Source: CAD feature listing. Evaluate the final solid. Frame: model axes, mm. A direction names the side the tool comes from. Coordinates: 2 decimals unless noted, no trailing zeros. Order: outer loops, then holes, each group sorted by start corner. A loop starts at its lowest first (then second) coordinate and runs counter-clockwise, first axis right, second up.
Item 1: Section A-A on x = -3. Return the cut outline in (y, z) (3 decimals), then the cut area to 3 significant figures.
Item 2: Section D-D on z = -3. State how many separate pieces and enclosed holes the cut face has, then the cut area to 3 significant figures.
Item 3: Ray query, line 1 (X direction, y = 0, z = 3.25) (3 decimals); line 2 (Y direction, x = -5, z = -0.5); line 3 (X direction, y = -4, z = 0.5). Return the intervals inside material, ascending.
Item 4: Mould query, pull axis Y, two halves, no side actions, for faces 1 (the flat face through (-8.5, 0, 0)), 2 (the flat face through (13.5, 0, 0)), 3 (the cylindrical face through (2.35, -6.23, -5.71)), 4 (the flat face through (20, -6.172, 0)). Classes: released by +Y, released by -Y, zero draft, split by the parting line, or undercut.
Item 5: Section C-C on y = 0. Return the cut outline in (x, z) (3 decimals).
Item 6: Reachability of faces 5 (the flat face through (20, 2.813, 0)), 6 (the flat face through (20, -2, 4.314)), 7 (the flat face through (20, -5, -4.569)), 8 (the flat face through (25.5, 6, -8)), 9 (the cylindrical face through (5.2, 2.15, -0.11)) from +Z, -Z, +X, -X, +Y, -Y: full face, straight path, thin tool, end or side. Return the list, or none.
Item 7: Contact query for flat-ended pins moving along their axis: P1, Ø10.5, axis at x = 0, y = 0, coming from the -Z side; P2, Ø7, axis at x = 22, y = -1, coming from the +Z side; P3, Ø4, axis at x = 2.5, z = -0.5, coming from the +Y side. Output: stop coordinate, or through.
Item 8: Section B-B on z = 2.5. Return the cut outline in (x, y) (3 decimals).
Autodesk Inventor part; units mm, degrees
ref_plane "YZ Plane" through (0, 0, 0) normal (1, 0, 0) x (0, 1, 0)
ref_plane "XZ Plane" through (0, 0, 0) normal (0, 1, 0) x (-1, 0, 0)
ref_plane "XY Plane" through (0, 0, 0) normal (0, 0, 1) x (1, 0, 0)
sketch "Sketch1" plane through (0, 0, 0) normal (1, 0, 0) x (0, 1, 0)
  circle A0 centre (0, 0) radius 8.45
  dimension "d0" = 16.9
extrude "Extrusion1" add sketch "Sketch1" along normal blind 13.5 and the other way blind 8.5
sketch "Sketch2" plane through (13.5, 0, 0) normal (1, 0, 0) x (0, 0, -1)
  circle A0 centre (0, 0) radius 7.725
  circle A1 centre (0, 0) radius 9.725
  dimension "d3" = 2
  dimension "d4" = 19.45
extrude "Extrusion2" cut sketch "Sketch2" against normal blind 21.5 contours A0
sketch "Sketch3" plane through (0, 0, 0) normal (0, 0, 1) x (1, 0, 0)
  circle A0 centre (0, 0) radius 5.625
  dimension "d7" = 11.25
extrude "Extrusion3" add sketch "Sketch3" along normal mid plane 18
sketch "Sketch4" plane through (0, 0, 0) normal (0, 0, 1) x (1, 0, 0)
  circle A0 centre (0, 0) radius 4.625
  dimension "d10" = 9.25
extrude "Extrusion5" cut sketch "Sketch4" along normal mid plane 100
sketch "Sketch5" plane through (13.5, 0, 0) normal (1, 0, 0) x (0, 0, -1)
  circle A0 centre (0, 0) radius 8.675
  dimension "d15" = 17.35
extrude "Extrusion6" add sketch "Sketch5" along normal blind 2
sketch "Sketch6" plane through (15.5, 0, 0) normal (1, 0, 0) x (0, 0, -1)
  arc A0 (1.0628, -4.9847) -> (6.3756, 23.0304) centre (-2.1717, 10.14) ccw
  spline S0 degree 4 poles (1.0628, -0.783) (3.325, -0.3237) (6.6509, 1.9196) (12.5543, 12.8577) (0.0955, 21.0445) (-3.8878, 23.6903) (2.1134, 24.7257) knots 0 0 0 0 0 0.38125 0.63125 1 1 1 1 1
  line L0 (-1.8785, -1.3802) -> (4.0041, -0.1858) construction
  arc A1 (-1.2523, -0.8951) -> (3.2382, 0.0167) centre (-0.4606, 6.7196) ccw construction
  spline S1 degree 2 poles (6.3756, 23.0304) (3.3857, 25.3291) (1.0628, 24.5204) knots 0 0 0 1 1 1
  line L1 (-6.8176, 23.1848) -> (11.0445, 26.2665) construction
  arc A2 (9.1477, 24.9445) -> (-4.5875, 22.5748) centre (6.4085, -0.169) ccw construction
  line L2 (-4.3138, 2.8134) -> (4.5692, 2.8134)
  line L3 (4.5692, -6.1723) -> (-4.3138, -6.1723)
  line L4 (-4.3138, -6.1723) -> (-4.3138, 2.8134)
  line L5 (4.5692, 2.8134) -> (4.5692, 1.038)
  line L6 (4.5692, -3.7804) -> (4.5692, -6.1723)
  point P0 (0, 0)
  point P1 (-0.6365, 21.8121)
  point P2 (1.0628, -0.783)
  point P3 (3.2364, 24.6304)
  point P4 (2.1134, 24.7257)
  point P5 (2.1133, 24.7254)
  point P6 (1.0633, 24.5166)
  dimension "d10" = 9.25
extrude "Extrusion7" add sketch "Sketch6" along normal blind 10 and the other way blind 2
sketch "Sketch7" plane through (-8.5, 0, 0) normal (-1, 0, 0) x (0, 0, 1)
  circle A0 centre (0, 0) radius 8.45
  circle A1 centre (0, 0) radius 11.1999
  dimension "d23" = 16.9
extrude "Extrusion8" cut sketch "Sketch7" against normal blind 17.75
properties part number "valve insert-mod"
Answer list:
1. outline: (-3.52, -7.682) - (-3.52, 7.682) arc R8.45 ccw to start; (3.52, -7.682) arc R8.45 ccw to (3.52, 7.682) - close; hole (-4.758, -6.086) - (-4.758, 6.086) arc R7.725 ccw to start; hole (4.758, -6.086) arc R7.725 ccw to (4.758, 6.086) - close
1. area: 58.5 mm2
2. separate pieces: 3
2. enclosed holes: 2
2. area: 269 mm2
3. line 1: x = -8.5 to -8, -5.625 to -4.625, 4.625 to 5.625, 13.5 to 25.5
3. line 2: y = -8.44 to -7.71, -2.58 to 2.58, 7.71 to 8.44
3. line 3: x = -8.5 to -8, -3.95 to -2.32, 2.32 to 3.95, 13.5 to 25.5
4. face 1: zero draft
4. face 2: undercut
4. face 3: split by the parting line
4. face 4: released by -Y
5. outline: (-8.5, -8.45) - (-4.625, -8.45) - (-4.625, 8.45) - (-8.5, 8.45) - close; (4.625, -8.45) - (13.5, -8.45) - (13.5, -9.507) - (25.5, -9.507) - (25.5, 4.314) - (15.5, 4.314) - (15.5, 8.675) - (13.5, 8.675) - (13.5, 8.45) - (4.625, 8.45) - close; hole (-8, -7.725) - (-5.625, -7.725) - (-5.625, 7.725) - (-8, 7.725) - close; hole (5.625, -7.725) - (13.5, -7.725) - (13.5, 7.725) - (5.625, 7.725) - close
6. face 5: +Z, +X
6. face 6: +Z, +X, +Y, -Y
6. face 7: -Z, +X, -Y
6. face 8: +Z, -Z, +X, +Y, -Y
6. face 9: none
7. P1: stops at z = -8.45
7. P2: stops at z = 4.31
7. P3: stops at y = 8.45
8. outline: (-8.5, -8.072) - (13.5, -8.072) - (13.5, -8.307) - (15.5, -8.307) - (15.5, -6.172) - (25.5, -6.172) - (25.5, 2.813) - (15.5, 2.813) - (15.5, 8.307) - (13.5, 8.307) - (13.5, 8.072) - (-8.5, 8.072) - close; circle Ø11.25 at (0, 0); hole (-8, -7.309) - (13.5, -7.309) - (13.5, 7.309) - (-8, 7.309) - close; hole circle Ø9.25 at (0, 0)
